Here's how the part is built. I have some questions about the finished solid (model axes, mm). Face numbers are marked on the shaded views. Coordinates: 2 decimals unless noted, no trailing zeros. Loops run counter-clockwise (first coordinate to the right, second up) from the corner with the lowest first, then second, coordinate; pieces in that order, holes last. Notation, with made-up numbers: M 46,60 L 60,60 A24 ccw 60,84 Z; hole C -31,16 d8. An arc over 180 degrees is marked long. Use one line per item in the form item = value. Start each with the question number.
(1) Please list where these lines run through material, in increasing order: L1, parallel to Z at x = -12.7, y = 4.25; L2, parallel to Z at x = -12.25, y = 0.5; L3, parallel to X at y = 0.5, z = -10.5.
(2) Imagine slicing it at A-A, the plane x = -12.7. Please give me the cut outline in (y, z), and give its area (3 significant figures).
(3) Imagine slicing it at B-B, the plane y = 5.5. Please give me the cut outline in (x, z).
(4) Thinking about a two-plate mould opening in Z: for the marked faces 1, 2 and 3, which applies, +Z half, -Z half, draft (parallel to the pull), parting line (faces both ways), or undercut?
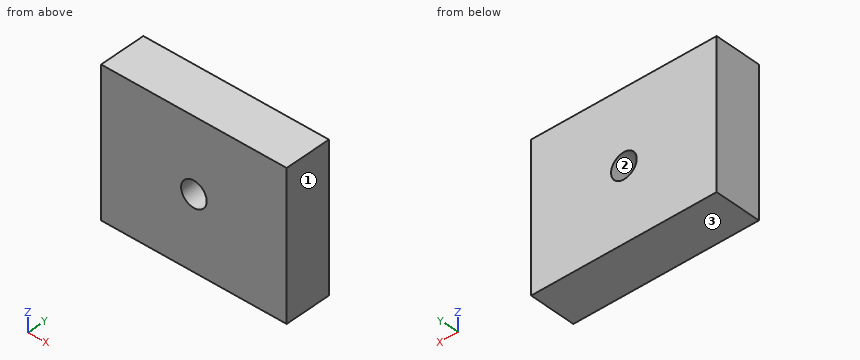
Autodesk Inventor part; units mm, degrees
ref_plane "YZ Plane" through (0, 0, 0) normal (1, 0, 0) x (0, 1, 0)
ref_plane "XZ Plane" through (0, 0, 0) normal (0, 1, 0) x (-1, 0, 0)
ref_plane "XY Plane" through (0, 0, 0) normal (0, 0, 1) x (1, 0, 0)
sketch "Sketch1" plane through (0, 0, 0) normal (0, 1, 0) x (-1, 0, 0)
  line L0 (0, 0) -> (25.4, 0)
  line L1 (25.4, 0) -> (25.4, -19.9898)
  line L2 (25.4, -19.9898) -> (0, -19.9898)
  line L3 (0, -19.9898) -> (0, 0)
  dimension "d0" = 25.4
  dimension "d1" = 19.9898
extrude "Extrusion1" add sketch "Sketch1" along normal blind 6.35
sketch "Sketch2" plane through (0, 6.35, 0) normal (0, 1, 0) x (1, 0, 0)
  line L0 (-25.4, 0) -> (0, 0)
  line L1 (0, 0) -> (0, 19.9898)
  line L2 (0, 19.9898) -> (-25.4, 19.9898)
  line L3 (-25.4, 19.9898) -> (-25.4, 0)
  point P0 (-12.7, 9.9949)
  dimension "d4" = 19.9898
  dimension "d5" = 25.4
  dimension "d6" = 12.7
  dimension "d7" = 9.9949
hole "Hole1" at (-12.7, 6.35, -9.9949) direction (0, -1, 0) diameter 3.5052 end through all
properties part number "SINGLE HOLE CONNECTOR"
Answer:
q1.L1 = -19.99 to -11.75, -8.24 to 0
q1.L2 = -19.99 to -11.69, -8.3 to 0
q1.L3 = -25.4 to -14.38, -11.02 to 0
q2.outline = M 0,-19.99 L 6.35,-19.99 L 6.35,-11.75 L 0,-11.75 Z; M 0,-8.24 L 6.35,-8.24 L 6.35,0 L 0,0 Z
q2.area = 105 mm²
q3.outline = M -25.4,-19.99 L 0,-19.99 L 0,0 L -25.4,0 Z; hole C -12.7,-9.99 d3.51
q4.face_1 = draft
q4.face_2 = undercut
q4.face_3 = -Z half
